Autodesk Inventor part; units mm, degrees
ref_plane "YZ Plane" through (0, 0, 0) normal (1, 0, 0) x (0, 1, 0)
ref_plane "XZ Plane" through (0, 0, 0) normal (0, 1, 0) x (-1, 0, 0)
ref_plane "XY Plane" through (0, 0, 0) normal (0, 0, 1) x (1, 0, 0)
sketch "Sketch1" plane through (0, 0, 0) normal (1, 0, 0) x (0, 1, 0)
  line L0 (0, 0) -> (15, 0)
  line L1 (15, 0) -> (15, -2)
  line L2 (15, -2) -> (0, -2)
  line L3 (0, -2) -> (0, 0)
  line L4 (0, 0) -> (2, 0)
  line L5 (2, 0) -> (2, -6)
  line L6 (2, -6) -> (0, -6)
  line L7 (0, -6) -> (0, 0)
  point P0 (0, -1)
  point P1 (1, 0)
  point P2 (1, -6)
  point P3 (2, -2)
  point P4 (0, -2)
  dimension "d0" = 15
  dimension "d1" = 2
  dimension "d2" = 2
  dimension "d3" = 6
extrude "Extrusion1" add sketch "Sketch1" along normal blind 200
properties part number "GuiderailRS3" material "Steel"
Read the model definition and answer for the solid it produces. Units are mm, in the model's axes. A direction names the side the tool comes from. Give positions to 0.01 mm unless a question says otherwise; leave off trailing zeros. Order: outer loops, then holes, each group sorted by start corner. A loop starts at its lowest first (then second) coordinate and runs counter-clockwise, first axis right, second up. Notation, with made-up numbers: (49.25, -15.5) -> (105.25, -15.5) arc R21 cw to (105.25, 3.5) -> close; hole circle Ø11 at (-25, 17). An arc over 180 degrees is marked (long way). One line per item, written item: value. Start each with the question number.
(1) Straight lines are drawn through the part: L1, parallel to Y at x = 182.5, z = -4.35; L2, parallel to Z at x = 126, y = 6.5. For each, find the intervals that lie inside material, in ascending order.
(2) A tool of negligible diameter and unlimited length cuts with its end or side. For faces 1 (the flat face through (99, 7, 0)), 2 (the flat face through (99, 9, -2)), from which of +Z, -Z, +X, -X, +Y, -Y can it reach the whole face along a straight path? Write none if from no direction.
(3) The part is cut by section C-C (z = -4.3). Determine the outline of the cut face in (x, y).
(4) The part is cut by section B-B (y = 12). Determine the outline of the cut face in (x, z), and give its area (3 significant figures).
(5) Flat-ended cylindrical pins translate along their axes: P1, Ø3, axis at x = 131.5, y = 9, coming from the -Z side; P2, Ø3, axis at x = 68.5, z = -4, coming from the +Y side. Find the tip coordinate at first contact, or state that the pin passes through.
(6) The part is cut by section A-A (x = 97). Determine the outline of the cut face in (y, z), and give its area (3 significant figures).
Taken from the geometry:
1. L1: 0 to 2
1. L2: -2 to 0
2. face 1: +Z, +X, -X, +Y, -Y
2. face 2: -Z, +X, -X, +Y
3. outline: (0, 0) -> (200, 0) -> (200, 2) -> (0, 2) -> close
4. outline: (0, -2) -> (200, -2) -> (200, 0) -> (0, 0) -> close
4. area: 400 mm^2
5. P1: z = -2
5. P2: y = 2
6. outline: (0, -6) -> (2, -6) -> (2, -2) -> (15, -2) -> (15, 0) -> (0, 0) -> close
6. area: 38.0 mm^2
